from build123d import *

# Parameters (mm, degrees)
SKETCH1_R           = 2.75
BOSS_EXTRUDE1_DEPTH = 2


with BuildPart() as part:
    # Sketch1 → Boss-Extrude1 (new body)
    with BuildSketch(Plane.XY):
        Polygon((5, 0), (38, 0), (75, 0), (80, 5), (80, 33), (75, 38), (39, 38), (38, 39), (38, 75), (33, 80), (5, 80), (0, 75), (0, 5), align=None)
        with Locations((9, 71)):
            Circle(SKETCH1_R, mode=Mode.SUBTRACT)
        with Locations((29, 71)):
            Circle(SKETCH1_R, mode=Mode.SUBTRACT)
        with Locations((29, 51)):
            Circle(SKETCH1_R, mode=Mode.SUBTRACT)
        with Locations((9, 51)):
            Circle(SKETCH1_R, mode=Mode.SUBTRACT)
        with Locations((51, 29)):
            Circle(SKETCH1_R, mode=Mode.SUBTRACT)
        with Locations((71, 29)):
            Circle(SKETCH1_R, mode=Mode.SUBTRACT)
        with Locations((71, 9)):
            Circle(SKETCH1_R, mode=Mode.SUBTRACT)
        with Locations((51, 9)):
            Circle(SKETCH1_R, mode=Mode.SUBTRACT)
    extrude(amount=BOSS_EXTRUDE1_DEPTH)


solid = part.part
The model under review builds one solid part; all positions refer to its coordinate system, in mm. A direction names the side the tool comes from. Give positions to 0.01 mm unless a question says otherwise; leave off trailing zeros. Write each loop counter-clockwise with the first axis right and the second up, starting at its lowest first coordinate (ties: lowest second). Pieces come first, ordered by that corner, then holes.
1. Wall thickness on L1, parallel to Y at x = 51, z = 1; L2, parallel to Y at x = 9, z = 1.15; L3, parallel to Y at x = 59, z = 0.8: over which ranges is each line inside the solid? List them lowest first.
2. Add section A-A, the plane y = 29. Write out the cut boundary in (x, z).
3. Tool access review of faces 4 (the cylindrical face through (48.253, 9.121, 0.986)), 5 (the flat face through (57, 38, 1)): name each direction out of +Z, -Z, +X, -X, +Y, -Y from which nothing blocks a thin tool from reaching the whole face with its end or side.
4. For P1, Ø0.6, axis at x = 62.5, z = 1.5, coming from the +Y side; P2, Ø3.5, axis at x = 29, y = 71, coming from the -Z side; P3, Ø1, axis at y = 49, z = 1, coming from the +X side, all flat-tipped, find the tip position at first contact; note any pin that passes through.
5. Add section D-D, the plane x = 43.5. Write out the cut boundary in (y, z).
6. Draft analysis for pull direction X (two halves, no side actions). For faces 1 (the flat face through (40, 0, 1)), 2 (the flat face through (78, 35, 1)), 3 (the cylindrical face through (8.642, 53.727, 0.986)), state which applies: +X half, -X half, draft (parallel to the pull), parting line (faces both ways), or undercut.
7. Add section C-C, the plane z = 1.2. Count the separate pieces of the cut face and the enclosed holes in it, plus the area to 3 significant figures.
Worked answers:
1. L1: y = 0 to 6.25, 11.75 to 26.25, 31.75 to 38
1. L2: y = 0 to 48.25, 53.75 to 68.25, 73.75 to 80
1. L3: y = 0 to 38
2. outline: (0, 0) - (48.25, 0) - (48.25, 2) - (0, 2) - close; (53.75, 0) - (68.25, 0) - (68.25, 2) - (53.75, 2) - close; (73.75, 0) - (80, 0) - (80, 2) - (73.75, 2) - close
3. face 4: +Z, -Z
3. face 5: +Z, -Z, +X, +Y
4. P1: stops at y = 38
4. P2: passes through
4. P3: stops at x = 38
5. outline: (0, 0) - (38, 0) - (38, 2) - (0, 2) - close
6. face 1: draft
6. face 2: +X half
6. face 3: undercut
7. separate pieces: 1
7. enclosed holes: 8
7. area: 4,380 mm2
